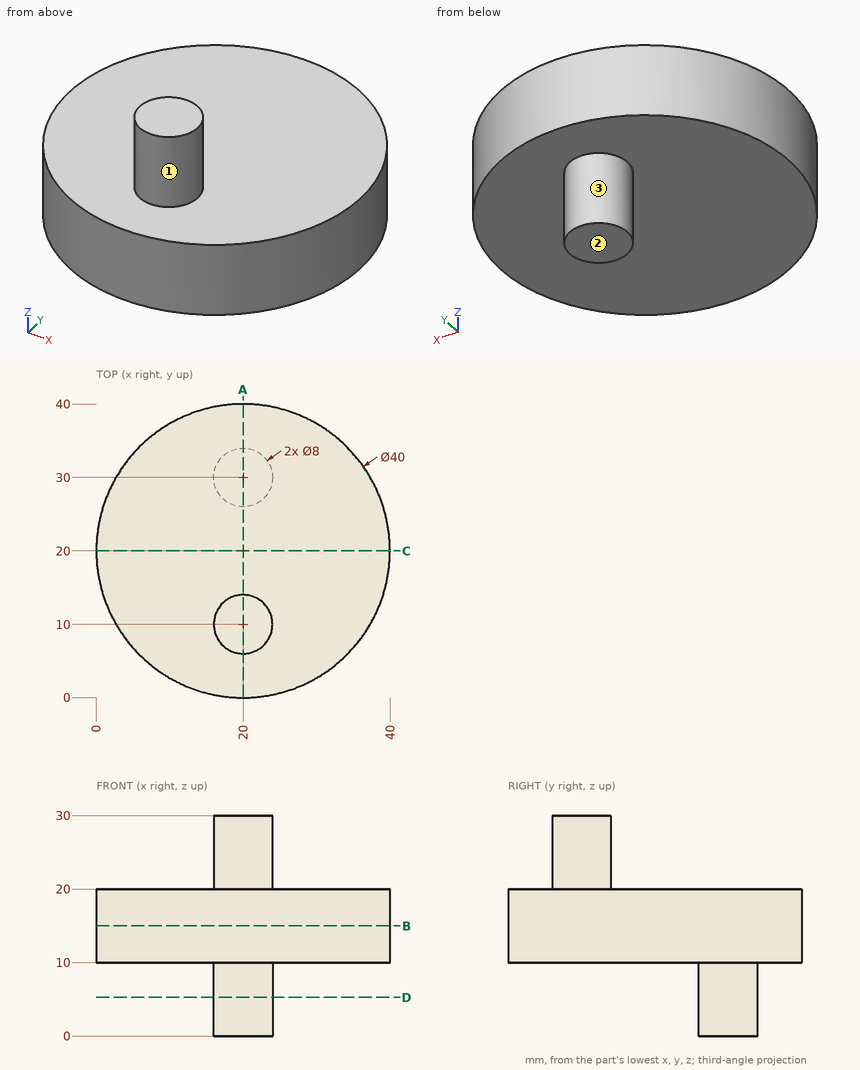
Job drawing, mm, ordinate dimensions from the low corner. One solid piece. A direction names the side the tool comes from. Give positions to 0.01 mm unless a question says otherwise; leave off trailing zeros. Order: outer loops, then holes, each group sorted by start corner. A loop starts at its lowest first (then second) coordinate and runs counter-clockwise, first axis right, second up. Notation, with made-up numbers: (36.25, 58.25) - (88.25, 58.25) arc R21 cw to (88.25, 96.25) - close; hole circle Ø5 at (20.5, 16.5). An arc over 180 degrees is marked (long way). Return JSON: item names as keys, results as strings.
1) Cut at B-B, the plane z = 15. Give the cut face in (x, y), plus the area to 3 significant figures.
Geometry says:
{"outline": "circle Ø40 at (20, 20)", "area": "1,260 mm²"}
2) 3-axis set-ups, long thin cutter, end or side, ignore diameter. For the marked faces 1, 2 and 3: which of +Z, -Z, +X, -X, +Y, -Y reach the whole face in a straight line?
Geometry says:
{"face 1": "+Z", "face 2": "-Z, +X, -X, +Y, -Y", "face 3": "-Z"}
3) Cut at C-C, the plane y = 20. Give the cut face in (x, z).
Geometry says:
{"outline": "(0, 10) - (40, 10) - (40, 20) - (0, 20) - close"}
4) Flat gauge pins, fed straight in: P1, Ø6, axis at x = 18.5, z = 9.5, coming from the +Y side; P2, Ø10, axis at y = 25, z = 6.5, coming from the +X side; P3, Ø6, axis at x = 14, y = 19, coming from the -Z side; P4, Ø1.5, axis at y = 12, z = 8, coming from the -X side. Where does each tip first touch, or does it go through?
Geometry says:
{"P1": "y = 40", "P2": "x = 39.95", "P3": "z = 10", "P4": "through"}
5) Probe line 1 (Z direction, x = 19.5, y = 10.5); line 2 (Z direction, x = 5.5, y = 25.5); line 3 (Y direction, x = 3.5, z = 13.25). List the from-to ranges inside material, lowest first. Write a range as from..to.
Geometry says:
{"line 1": "10..30", "line 2": "10..20", "line 3": "8.7..31.3"}
6) Cut at A-A, the plane x = 20. Give the cut face in (y, z), plus the area to 3 significant figures.
Geometry says:
{"outline": "(0, 10) - (26, 10) - (26, 0) - (34, 0) - (34, 10) - (40, 10) - (40, 20) - (14, 20) - (14, 30) - (6, 30) - (6, 20) - (0, 20) - close", "area": "560 mm²"}
7) Cut at D-D, the plane z = 5.25. Give the cut face in (x, y), plus the area to 3 significant figures.
Geometry says:
{"outline": "circle Ø8 at (20, 30)", "area": "50.3 mm²"}
